For this review, take the finished solid that the model builds, in its own axes (mm). Coordinates: 2 decimals unless noted, no trailing zeros. Write each loop counter-clockwise with the first axis right and the second up, starting at its lowest first coordinate (ties: lowest second). Pieces come first, ordered by that corner, then holes.
1) We need section A-A on x = 179.5. Write out the cut boundary in (y, z).
2) To check wall thickness, follow line 1 along X through (y, z) = (27, 0.85); line 2 along Y through (x, z) = (196, 0.3); line 3 along X through (y, z) = (20, 1.7). State the ranges of each line that lie inside material, in increasing order.
3) Insertion check: P1, Ø1.5, axis at x = 55, z = 1, coming from the -Y side; P2, Ø1, axis at x = 110.5, z = 0.5, coming from the +Y side; P3, Ø0.9, axis at y = 14, z = 1, coming from the +X side. Each pin has a flat end and moves straight along its axis. Give the tip position at first contact, or say it passes through.
4) We need section C-C on x = 239. Write out the cut boundary in (y, z), then the cut area to 3 significant figures.
5) We need section B-B on z = 2.15. Give the number of separate pieces and of enclosed holes in the cut face, then the cut area to 3 significant figures.
Autodesk Inventor part; units mm, degrees
ref_plane "YZ Plane" through (0, 0, 0) normal (1, 0, 0) x (0, 1, 0)
ref_plane "XZ Plane" through (0, 0, 0) normal (0, 1, 0) x (-1, 0, 0)
ref_plane "XY Plane" through (0, 0, 0) normal (0, 0, 1) x (1, 0, 0)
sketch "Sketch1" plane through (0, 0, 0) normal (0, 0, 1) x (1, 0, 0)
  line L0 (0, 0) -> (300, 0)
  line L1 (300, 0) -> (300, 16)
  line L2 (300, 16) -> (0, 16)
  line L3 (0, 16) -> (0, 0)
  line L4 (0, 0) -> (22.0483, 0)
  line L5 (10, 0) -> (29.5, 0)
  line L6 (29.5, 0) -> (29.5, -15)
  line L7 (29.5, -15) -> (10, -15)
  line L8 (10, -15) -> (10, 0)
  point P0 (0, 8)
  dimension "d2" = 19.5
  dimension "d3" = 15
  dimension "d4" = 10
  dimension "d5" = 16
  dimension "d8" = 300
extrude "Extrusion1" add sketch "Sketch1" along normal blind 3
sketch "Sketch2" plane through (0, 0, 3) normal (0, 0, 1) x (1, 0, 0)
  line L0 (0, 16) -> (0, 0)
  line L1 (0, 16) -> (0, 36)
  line L2 (300, 0) -> (300, 16)
  line L3 (340, 16) -> (340, 36)
  line L4 (340, 36) -> (0, 36)
  line L5 (300, 16) -> (0, 16)
  line L6 (50, 16) -> (50, 30)
  line L7 (50, 30) -> (210, 30)
  line L8 (210, 30) -> (210, 16)
  line L9 (40, 36) -> (36, 56)
  line L10 (36, 56) -> (42, 56)
  line L11 (42, 56) -> (46, 36)
  circle A0 centre (330, 30) radius 2.1
  circle A1 centre (330, 20.6) radius 2.1
  line L12 (340, 16) -> (300, 16)
  line L13 (301, 36) -> (316, 36)
  line L14 (316, 36) -> (316, 48)
  line L15 (316, 48) -> (301, 48)
  line L16 (301, 48) -> (301, 36)
  circle A2 centre (308.5, 43) radius 2.075
  line L17 (36, 56) -> (30, 56)
  line L18 (30, 56) -> (31.1, 50.5)
  line L19 (31.1, 50.5) -> (37.1, 50.5)
  point P0 (308.5, 48)
  point P1 (316, 36)
  dimension "d44" = 20
  dimension "d45" = 160
  dimension "d46" = 50
  dimension "d47" = 14
  dimension "d48" = 20
  dimension "d49" = 6
  dimension "d50" = 4
  dimension "d51" = 40
  dimension "d83" = 4.2
  dimension "d84" = 4.2
  dimension "d85" = 6
  dimension "d86" = 9.4
  dimension "d87" = 10
  dimension "d99" = 40
  dimension "d107" = 7
  dimension "d108" = 15
  dimension "d109" = 12
  dimension "d110" = 24
  dimension "d111" = 4.15
  dimension "d112" = 6
  dimension "d114" = 5.5
extrude "Extrusion2" add sketch "Sketch2" against normal blind 3 contours L1 L4 L3 L12 L5 L8 L7 L6 | L9 L10 L11 L4 | L19 L18 L17 L9 | L16 L15 L14 L4
sketch "Sketch3" plane through (0, 0, 3) normal (0, 0, 1) x (1, 0, 0)
  circle A0 centre (16.5, -6.5) radius 2.1
  circle A1 centre (24.5, -7) radius 2.1
  line L0 (29.5, 0) -> (300, 0)
  line L1 (29.5, -15) -> (29.5, 0)
  point P0 (0, 0)
  dimension "d75" = 4.2
  dimension "d76" = 6.5
  dimension "d77" = 4.2
  dimension "d78" = 7
  dimension "d79" = 5
  dimension "d80" = 8
extrude "Extrusion3" cut sketch "Sketch3" against normal blind 3
sketch "Sketch4" plane through (0, 0, 3) normal (0, 0, 1) x (1, 0, 0)
  line L0 (29.5, 0) -> (300, 0)
  circle A0 centre (41, 18) radius 2.6
  line L1 (340, 36) -> (46, 36)
  line L2 (38.4, 28.1) -> (43.6, 28.1)
  line L3 (43.6, 28.1) -> (43.6, 7.9)
  line L4 (43.6, 7.9) -> (38.4, 7.9)
  line L5 (38.4, 7.9) -> (38.4, 28.1)
  line L6 (38.4, 28.1) -> (43.6, 7.9) construction
  line L7 (43.6, 28.1) -> (38.4, 7.9) construction
  point P0 (0, 0)
  point P1 (43.6, 18)
  point P2 (38.4, 18)
  dimension "d95" = 18
  dimension "d96" = 5.2
  dimension "d100" = 5
  dimension "d101" = 20.2
extrude "Extrusion4" cut sketch "Sketch4" against normal blind 3
sketch "Sketch5" plane through (0, 0, 3) normal (0, 0, 1) x (1, 0, 0)
  line L0 (29.5, 0) -> (300, 0)
  line L1 (340, 36) -> (340, 16)
  arc A0 (300, 0) -> (340, 16) centre (300, 58) ccw
  line L2 (300, 0) -> (300, 16)
  line L3 (300, 0) -> (300, 16)
  line L4 (300, 16) -> (340, 16)
  point P0 (0, 0)
extrude "Extrusion5" add sketch "Sketch5" against normal blind 3
properties part number "Middle_bar"
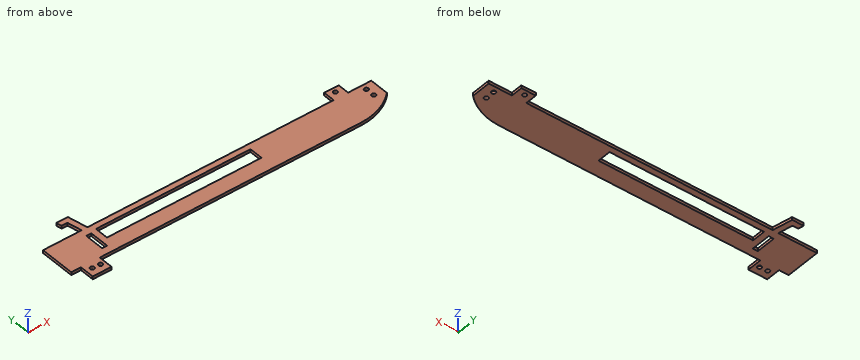
Result:
1. outline: (0, 0) - (16, 0) - (16, 3) - (0, 3) - close; (30, 0) - (36, 0) - (36, 3) - (30, 3) - close
2. line 1: x = 0 to 38.4, 43.6 to 50, 210 to 340
2. line 2: y = 0 to 16, 30 to 36
2. line 3: x = 0 to 38.4, 43.6 to 50, 210 to 327.99, 332.01 to 340
3. P1: stops at y = 0
3. P2: stops at y = 36
3. P3: stops at x = 338.31
4. outline: (0, 0) - (36, 0) - (36, 3) - (0, 3) - close
4. area: 108 mm2
5. separate pieces: 1
5. enclosed holes: 7
5. area: 10,300 mm2
